For this review, take the finished solid that the model builds, in its own axes (mm). A direction names the side the tool comes from. Give positions to 0.01 mm unless a question says otherwise; leave off trailing zeros. Order: outer loops, then holes, each group sorted by start corner. A loop starts at its lowest first (then second) coordinate and runs counter-clockwise, first axis right, second up. Notation, with made-up numbers: (67, -8) -> (88, -8) arc R17 cw to (88, 8) -> close; hole circle Ø10 at (-11.75, 30.25). An arc over 180 degrees is marked (long way). One line per item, written item: value. Start each with the question number.
from build123d import *

# Parameters (mm, degrees)
SKETCH1_W                = 57
SKETCH1_H                = 57
EXTRUDE1_DEPTH           = 76
F_5_0_5_DIAMETER_HOLE1_D = 5
SKETCH6_R                = 4
SKETCH6_R_2              = 2.5
EXTRUDE4_DEPTH           = 71
FILLET1_R                = 5
EXTRUDE5_DEPTH           = 25
EXTRUDE5_DEPTH_BACK      = 101
SKETCH7_R                = 3
SKETCH8_R                = 15
EXTRUDE6_DEPTH           = 3
FILLET2_R                = 1


with BuildPart() as part:
    # Sketch1 → Extrude1 (new body)
    with BuildSketch(Plane(origin=(0, 0, 0), x_dir=(1, 0, 0), z_dir=(0, 1, 0))):
        Rectangle(SKETCH1_W, SKETCH1_H)
    extrude(amount=EXTRUDE1_DEPTH)

    # Ø5.0 (5) Diameter Hole1 (through all)
    with Locations(Plane.XZ):
        with Locations((-23.5, 23.5), (23.5, 23.5), (23.5, -23.5), (-23.5, -23.5)):
            Hole(F_5_0_5_DIAMETER_HOLE1_D / 2)

    # Sketch6 → Extrude4 (cut)
    # profile 1 of 12: a face of its own
    with BuildSketch(Plane(origin=(0, 76, 0), x_dir=(1, 0, 0), z_dir=(0, 1, 0))):
        Polygon((-28.5, 28.5), (-19.5, 28.5), (-19.5, 32.511741208), (-33.908905561, 32.511741208), (-33.908905561, 19.5), (-28.5, 19.5), align=None)
    # profile 2 of 12: a face of its own
    with BuildSketch(Plane(origin=(0, 76, 0), x_dir=(1, 0, 0), z_dir=(0, 1, 0))):
        with BuildLine():
            ThreePointArc((-23.5, 19.5), (-26.328427125, 26.328427125), (-19.5, 23.5))
            Line((-19.5, 23.5), (-19.5, 28.5))
            Line((-19.5, 28.5), (-28.5, 28.5))
            Line((-28.5, 28.5), (-28.5, 19.5))
            Line((-28.5, 19.5), (-23.5, 19.5))
        make_face()
    # profile 3 of 12: a face of its own
    with BuildSketch(Plane(origin=(0, 76, 0), x_dir=(1, 0, 0), z_dir=(0, 1, 0))):
        with Locations((-23.5, 23.5)):
            Circle(SKETCH6_R)
        with Locations(Location((-23.5, 23.5, 0), (0, 0, 90))):
            Circle(SKETCH6_R_2, mode=Mode.SUBTRACT)
    # profile 4 of 12: a face of its own
    with BuildSketch(Plane(origin=(0, 76, 0), x_dir=(1, 0, 0), z_dir=(0, 1, 0))):
        Polygon((19.5, 36.471560472), (19.5, 28.5), (28.5, 28.5), (28.5, 19.5), (41.168352552, 19.5), (41.168352552, 36.471560472), align=None)
    # profile 5 of 12: a face of its own
    with BuildSketch(Plane(origin=(0, 76, 0), x_dir=(1, 0, 0), z_dir=(0, 1, 0))):
        with BuildLine():
            Line((28.5, 28.5), (19.5, 28.5))
            Line((19.5, 28.5), (19.5, 23.5))
            ThreePointArc((19.5, 23.5), (23.5, 27.5), (27.5, 23.5))
            ThreePointArc((27.5, 23.5), (26.328427125, 20.671572875), (23.5, 19.5))
            Line((23.5, 19.5), (28.5, 19.5))
            Line((28.5, 19.5), (28.5, 28.5))
        make_face()
    # profile 6 of 12: a face of its own
    with BuildSketch(Plane(origin=(0, 76, 0), x_dir=(1, 0, 0), z_dir=(0, 1, 0))):
        with Locations((23.5, 23.5)):
            Circle(SKETCH6_R)
        with Locations(Location((23.5, 23.5, 0), (0, 0, 90))):
            Circle(SKETCH6_R_2, mode=Mode.SUBTRACT)
    # profile 7 of 12: a face of its own
    with BuildSketch(Plane(origin=(0, 76, 0), x_dir=(1, 0, 0), z_dir=(0, 1, 0))):
        with Locations((23.5, -23.5)):
            Circle(SKETCH6_R)
        with Locations(Location((23.5, -23.5, 0), (0, 0, 90))):
            Circle(SKETCH6_R_2, mode=Mode.SUBTRACT)
    # profile 8 of 12: a face of its own
    with BuildSketch(Plane(origin=(0, 76, 0), x_dir=(1, 0, 0), z_dir=(0, 1, 0))):
        with BuildLine():
            Line((28.5, -28.5), (28.5, -19.5))
            Line((28.5, -19.5), (23.5, -19.5))
            ThreePointArc((23.5, -19.5), (26.328427125, -20.671572875), (27.5, -23.5))
            ThreePointArc((27.5, -23.5), (23.5, -27.5), (19.5, -23.5))
            Line((19.5, -23.5), (19.5, -28.5))
            Line((19.5, -28.5), (28.5, -28.5))
        make_face()
    # profile 9 of 12: a face of its own
    with BuildSketch(Plane(origin=(0, 76, 0), x_dir=(1, 0, 0), z_dir=(0, 1, 0))):
        Polygon((44.252209519, -19.5), (28.5, -19.5), (28.5, -28.5), (19.5, -28.5), (19.5, -40.050429997), (44.252209519, -40.050429997), align=None)
    # profile 10 of 12: a face of its own
    with BuildSketch(Plane(origin=(0, 76, 0), x_dir=(1, 0, 0), z_dir=(0, 1, 0))):
        Polygon((-28.5, -28.5), (-28.5, -19.5), (-37.670786859, -19.5), (-37.670786859, -37.828231874), (-19.5, -37.828231874), (-19.5, -28.5), align=None)
    # profile 11 of 12: a face of its own
    with BuildSketch(Plane(origin=(0, 76, 0), x_dir=(1, 0, 0), z_dir=(0, 1, 0))):
        with BuildLine():
            Line((-23.5, -19.5), (-28.5, -19.5))
            Line((-28.5, -19.5), (-28.5, -28.5))
            Line((-28.5, -28.5), (-19.5, -28.5))
            Line((-19.5, -28.5), (-19.5, -23.5))
            ThreePointArc((-19.5, -23.5), (-26.328427125, -26.328427125), (-23.5, -19.5))
        make_face()
    # profile 12 of 12: a face of its own
    with BuildSketch(Plane(origin=(0, 76, 0), x_dir=(1, 0, 0), z_dir=(0, 1, 0))):
        with Locations((-23.5, -23.5)):
            Circle(SKETCH6_R)
        with Locations(Location((-23.5, -23.5, 0), (0, 0, 90))):
            Circle(SKETCH6_R_2, mode=Mode.SUBTRACT)
    extrude(amount=-EXTRUDE4_DEPTH, mode=Mode.SUBTRACT)

    # Fillet1
    fillet1_edges = [part.edges().sort_by_distance(p)[0] for p in [
        (-28.5, 2.5, 28.5),
        (-28.5, 2.5, -28.5),
        (28.5, 2.5, -28.5),
        (28.5, 2.5, 28.5),
    ]]
    fillet(fillet1_edges, radius=FILLET1_R)



with BuildPart() as body_2:
    # Sketch7 → Extrude5 (new, two sides: drawn at the far end of the back side and taken through both)
    with BuildSketch(Plane(origin=(0, 76, 0), x_dir=(1, 0, 0), z_dir=(0, 1, 0)).offset(-EXTRUDE5_DEPTH_BACK)):
        with Locations(Location((0, 0, 0), (0, 0, 270))):
            Circle(SKETCH7_R)
    extrude(amount=EXTRUDE5_DEPTH + EXTRUDE5_DEPTH_BACK)


with BuildPart() as part_1:
    add(part.part)

    add(body_2.part)  # Extrude6 merges body 2
    # Sketch8 → Extrude6 (add)
    with BuildSketch(Plane.XZ):
        with Locations(Location((0, 0, 0), (0, 0, 270))):
            Circle(SKETCH8_R)
    extrude(amount=EXTRUDE6_DEPTH)

    # Fillet2
    fillet2_edges = [part_1.edges().sort_by_distance(p)[0] for p in [
        (-28.5, 40.5, 19.5),
        (0, 76, 28.5),
        (-19.5, 40.5, 28.5),
        (-19.5, 76, 26),
        (-20.671572875, 76, 20.671572875),
        (-26, 76, 19.5),
        (-28.5, 76, 0),
        (-28.5, 40.5, -19.5),
        (-19.5, 40.5, -28.5),
        (-19.5, 76, -26),
        (-26, 76, -19.5),
        (-20.671572875, 76, -20.671572875),
        (0, 76, -28.5),
        (19.5, 76, -26),
        (26, 76, -19.5),
        (20.671572875, 76, -20.671572875),
        (19.5, 40.5, -28.5),
        (28.5, 40.5, -19.5),
        (19.5, 40.5, 28.5),
        (28.5, 76, 0),
        (26, 76, 19.5),
        (19.5, 76, 26),
        (20.671572875, 76, 20.671572875),
        (28.5, 40.5, 19.5),
    ]]
    fillet(fillet2_edges, radius=FILLET2_R)


solid = part_1.part
Q1. Mouldability with a two-part tool opening along X and no side actions: class faces 1 (the cylindrical face through (25.34, 2.53, 25.19)), 2 (the flat face through (0, 37, 28.5)), 3 (the flat face through (19.5, 40, -26)) as pulls with the +X half, pulls with the -X half, needs draft (parallel to the pull), parting line crosses it, or undercut.
Q2. Take a section at C-C (z = 0). State the section outline as (x, y) points.
Q3. For line 1 along Z through (x, y) = (23.5, 3); line 2 along X through (y, z) = (2, 23); line 3 along Y through (x, z) = (12, 14), list the stretches that pass through material, from the lowest coordinate up.
Q4. Take a section at B-B (x = 0). State the section outline as (y, z) points.
Q5. Take a section at D-D (z = 7.5). State the section outline as (x, y) points, and give its area (3 significant figures).
Q6. For faces 4 (the flat face through (25, 40, -19.5)), 5 (the flat face through (-25, 40, 19.5)), 6 (the cylindrical face through (-21.66, 2.53, 25.19)), 7 (the flat face through (0, 37, -28.5)), 8 (the flat face through (-13, 0, -13)), list the 3-axis set-ups (+Z, -Z, +X, -X, +Y, -Y) from which the entire face can be reached by the end or side of a thin tool; tool diameter is ignored.
Q7. For pin 1 Ø11 at (x, z) = (22, 22.5) entering from +Y; pin 2 Ø2 at (x, z) = (-22, 22.5) entering from -Y; pin 3 Ø2 at (x, y) = (26.5, 49.5) entering from -Z; pin 4 Ø3 at (x, z) = (-23.5, -23.5) entering from -Y, all flat-tipped, find the tip position at first contact; note any pin that passes through.
Q8. Take a section at A-A (y = 73). State the section outline as (x, z) points.
Answers below:
1. face 1: undercut
1. face 2: needs draft
1. face 3: pulls with the +X half
2. outline: (-28.5, 0) -> (-15, 0) -> (-15, -3) -> (-3, -3) -> (-3, -25) -> (3, -25) -> (3, -3) -> (15, -3) -> (15, 0) -> (28.5, 0) -> (28.5, 75) arc R1 ccw to (27.5, 76) -> (3, 76) -> (3, 101) -> (-3, 101) -> (-3, 76) -> (-27.5, 76) arc R1 ccw to (-28.5, 75) -> close
3. line 1: z = -28.5 to -26, -21 to 21, 26 to 28.5
3. line 2: x = -28.5 to -25.95, -21.05 to 21.05, 25.95 to 28.5
3. line 3: y = 0 to 76
4. outline: (-25, -3) -> (-3, -3) -> (-3, -15) -> (0, -15) -> (0, -28.5) -> (75, -28.5) arc R1 ccw to (76, -27.5) -> (76, -3) -> (101, -3) -> (101, 3) -> (76, 3) -> (76, 27.5) arc R1 ccw to (75, 28.5) -> (0, 28.5) -> (0, 15) -> (-3, 15) -> (-3, 3) -> (-25, 3) -> close
5. outline: (-28.5, 0) -> (-12.99, 0) -> (-12.99, -3) -> (12.99, -3) -> (12.99, 0) -> (28.5, 0) -> (28.5, 75) arc R1 ccw to (27.5, 76) -> (-27.5, 76) arc R1 ccw to (-28.5, 75) -> close
5. area: 4,410 mm²
6. face 4: -Z, +X, +Y
6. face 5: +Z, -X, +Y
6. face 6: +Y, -Y
6. face 7: -Z, +X, -X, +Y, -Y
6. face 8: -Y
7. pin 1: stops at y = 76
7. pin 2: stops at y = 0
7. pin 3: stops at z = -19.5
7. pin 4: passes through
8. outline: (-28.5, -18.5) arc R1 ccw to (-27.5, -19.5) -> (-23.5, -19.5) arc R4 cw to (-19.5, -23.5) -> (-19.5, -27.5) arc R1 ccw to (-18.5, -28.5) -> (18.5, -28.5) arc R1 ccw to (19.5, -27.5) -> (19.5, -23.5) arc R4 cw to (23.5, -19.5) -> (27.5, -19.5) arc R1 ccw to (28.5, -18.5) -> (28.5, 18.5) arc R1 ccw to (27.5, 19.5) -> (23.5, 19.5) arc R4 cw to (19.5, 23.5) -> (19.5, 27.5) arc R1 ccw to (18.5, 28.5) -> (-18.5, 28.5) arc R1 ccw to (-19.5, 27.5) -> (-19.5, 23.5) arc R4 cw to (-23.5, 19.5) -> (-27.5, 19.5) arc R1 ccw to (-28.5, 18.5) -> close
